Check sheet for the modelled part. Datum: model origin and axes. Units: mm. A direction names the side the tool comes from. Coordinates: 2 decimals unless noted, no trailing zeros. Loops run counter-clockwise (first coordinate to the right, second up) from the corner with the lowest first, then second, coordinate; pieces in that order, holes last.
```python
from build123d import *

# Parameters (mm, degrees)
F2_SIZE  = 0.5
F3_SIZE2 = 0.8660254038
F3_SIZE  = 1.5
F4_R     = 0.5
F5_W     = 5
F5_H     = 2.7889910041
F5_H_2   = 4.1100917986
F6_DEPTH = 12.5


with BuildPart() as f1:
    # F0 (on Front) → F1 (revolve)
    with BuildSketch(Plane.XZ):
        with BuildLine():
            Line((0, 5), (0, 2.5))
            Line((0, 2.5), (38, 2.5))
            Line((38, 2.5), (38, 5))
            Line((38, 5), (35.4364916731, 5))
            ThreePointArc((35.4364916731, 5), (33.5, 5.5), (31.5635083269, 5))
            Line((31.5635083269, 5), (18, 5))
            Line((18, 5), (18, 7.5))
            Line((18, 7.5), (15, 7.5))
            Line((15, 7.5), (15, 5))
            Line((15, 5), (0, 5))
        make_face()
    revolve(axis=Axis((21.8194629997, 0, 0), (1, 0, 0)))

    # F2
    f2_edges = [f1.edges().sort_by_distance(p)[0] for p in [
        (0, 0, -5),
        (18, 0, -7.5),
        (15, 0, -7.5),
        (0, 0, -2.5),
        (38, 0, -2.5),
    ]]
    chamfer(f2_edges, length=F2_SIZE)

    # F3
    f3_edges = [f1.edges().sort_by_distance(p)[0] for p in [
        (38, 0, -5),
    ]]
    f3_side = f1.faces().sort_by_distance((36.718246, 0, -5))[0]
    chamfer(f3_edges, length=F3_SIZE, length2=F3_SIZE2, reference=f3_side)

    # F4
    f4_edges = [f1.edges().sort_by_distance(p)[0] for p in [
        (18, 0, -5),
        (15, 0, -5),
    ]]
    fillet(f4_edges, radius=F4_R)

    # F5 (on Front) → F6 (cut, symmetric)
    with BuildSketch(Plane.XZ):
        with Locations((16.6406241506, 7.894495502)):
            Rectangle(F5_W, F5_H)
        with Locations((16.6406241506, -8.5550458993)):
            Rectangle(F5_W, F5_H_2)
    extrude(amount=F6_DEPTH, both=True, mode=Mode.SUBTRACT)


solid = f1.part
```
1) Section check A-A on x = 25.5. Enter the section's corners in (y, z).
Answer sheet:
outline: circle Ø10 at (0, 0); hole circle Ø5 at (0, 0)
2) Mould release check, pull along Y, two halves, no side actions. Record for faces 4 (the flat face through (16, 0, 6.5)), 5 (the conical face through (15.135, -7.134, 0.119)), 6 (the cylindrical face through (19.26, 2.44, -0.54)): +Y half, -Y half, draft (parallel to the pull), parting line (faces both ways), or undercut.
Answer sheet:
face 4: draft
face 5: -Y half
face 6: undercut
3) Scan lines: line 1 (Z direction, x = 14, y = 0); line 2 (Y direction, x = 16, z = 0). Record each from-to range of solid material in increasing order.
Answer sheet:
line 1: z = -5 to -2.5, 2.5 to 5
line 2: y = -7.5 to -2.5, 2.5 to 7.5
4) Depth check by flat-ended pin: pin 1 (3 mm diameter, centred on x = 21, z = 5, fed in from +Y); pin 2 (4 mm diameter, centred on x = 8.5, y = -3, fed in from +Z); pin 3 (2 mm diameter, centred on x = 8, z = 0, fed in from -Y). Enter the tip coordinate at first touch or a pass-through.
Answer sheet:
pin 1: stops at y = 3.57
pin 2: stops at z = 4.9
pin 3: stops at y = -5
5) Set-up check for faces 1 (the flat face through (18, -5, -3)), 2 (the cylindrical face through (24.94, 4.88, -1.08)), 3 (the flat face through (15, -5, 3)): record each of +Z, -Z, +X, -X, +Y, -Y from which the full face is reachable in a straight line by a thin tool's end or side.
Answer sheet:
face 1: +X
face 2: none
face 3: -X
